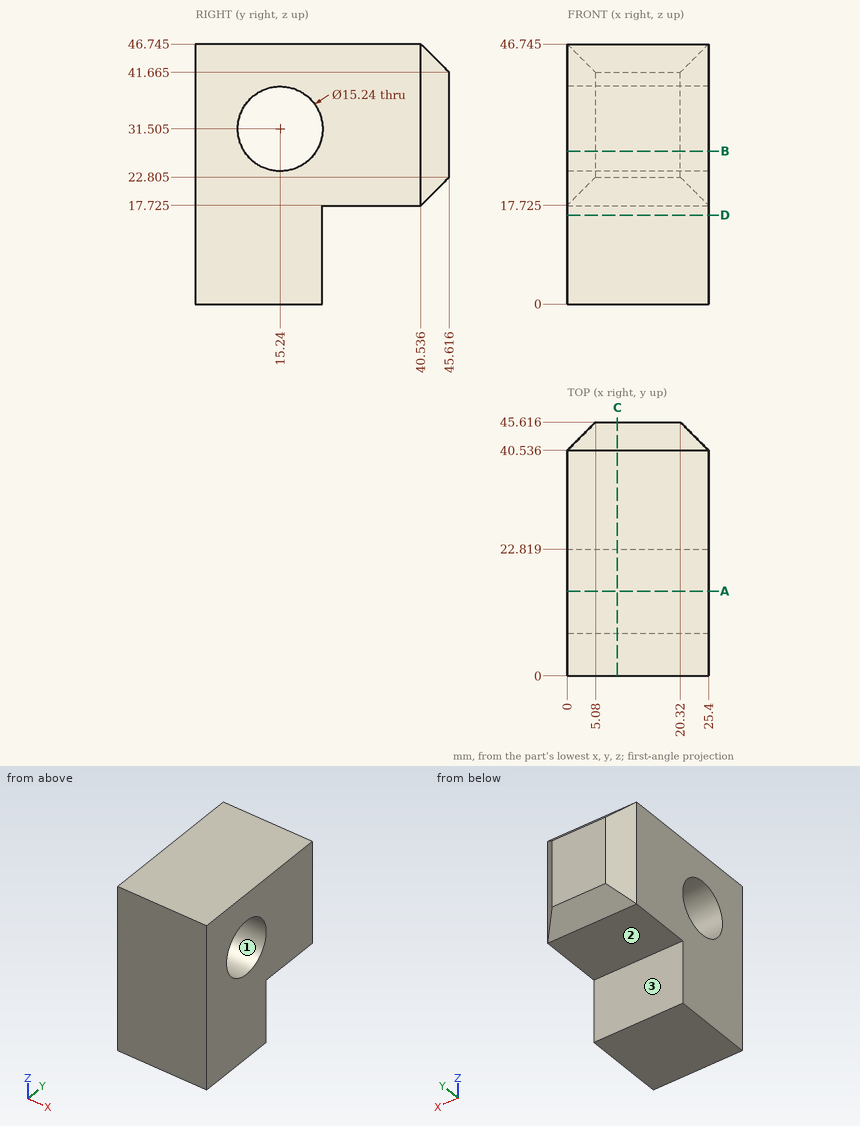
Print and shaded views of the part. All mm, measured from the part's lowest x, y and z. Round coordinates to 2 decimals unless told otherwise and drop trailing zeros. Write each loop counter-clockwise with the first axis right and the second up, starting at its lowest first coordinate (ties: lowest second). Pieces come first, ordered by that corner, then holes. Notation, with made-up numbers: (33.25, -24.75) - (42.25, -24.75) arc R32 ccw to (42.25, 4.25) - close; hole circle Ø11 at (-30.75, -19). An arc over 180 degrees is marked (long way). Write each question's results on one line, items separated by ' | '. Start each with the question number.
Item 1: Saw through at D-D (z = 16). Write the cut outline in (x, y), and give its area (3 significant figures).
Item 2: Wall check: L1, parallel to Y at x = 13, z = 31.5; L2, parallel to Z at x = 10.75, y = 35 (1 decimal); L3, parallel to Z at x = 15, y = 15.24 (1 decimal). Give the ranges that are in metal, low to high. Write a range as [from, to].
Item 3: Drop flat-ended pins along their axis: P1, Ø9, axis at y = 15.24, z = 31.51, coming from the +X side; P2, Ø12, axis at x = 22.5, z = 16.5, coming from the +Y side; P3, Ø12, axis at x = 20.5, z = 37, coming from the -Y side; P4, Ø9, axis at x = 11.5, y = 32.5, coming from the -Z side (1 decimal). Give the stop position or say it passes through.
Item 4: Saw through at B-B (z = 27.5). Write the cut outline in (x, y).
Item 5: Saw through at A-A (y = 15.24). Write the cut outline in (x, z) (1 decimal), and give its area (3 significant figures).
Item 6: Saw through at C-C (x = 9). Write the cut outline in (y, z) (1 decimal).
Item 7: Mould opens along Y. For the marked faces 1, 2 and 3 say: pulls with the +Y half, pulls with the -Y half, needs draft (parallel to the pull), parting line crosses it, or undercut.
Results are:
1) outline: (0, 0) - (25.4, 0) - (25.4, 22.82) - (0, 22.82) - close | area: 580 mm²
2) L1: y = [0, 7.62], [22.86, 45.62] | L2: z = [17.7, 46.7] | L3: z = [0, 23.9], [39.1, 46.7]
3) P1: passes through | P2: stops at y = 45.08 | P3: stops at y = 0 | P4: stops at z = 17.7
4) outline: (0, 0) - (25.4, 0) - (25.4, 8.76) - (0, 8.76) - close; (0, 21.72) - (25.4, 21.72) - (25.4, 40.54) - (20.32, 45.62) - (5.08, 45.62) - (0, 40.54) - close
5) outline: (0, 0) - (25.4, 0) - (25.4, 23.9) - (0, 23.9) - close; (0, 39.1) - (25.4, 39.1) - (25.4, 46.7) - (0, 46.7) - close | area: 800 mm²
6) outline: (0, 0) - (22.8, 0) - (22.8, 17.7) - (40.5, 17.7) - (45.6, 22.8) - (45.6, 41.7) - (40.5, 46.7) - (0, 46.7) - close; hole circle Ø15.2 at (15.2, 31.5)
7) face 1: undercut | face 2: needs draft | face 3: pulls with the +Y half
